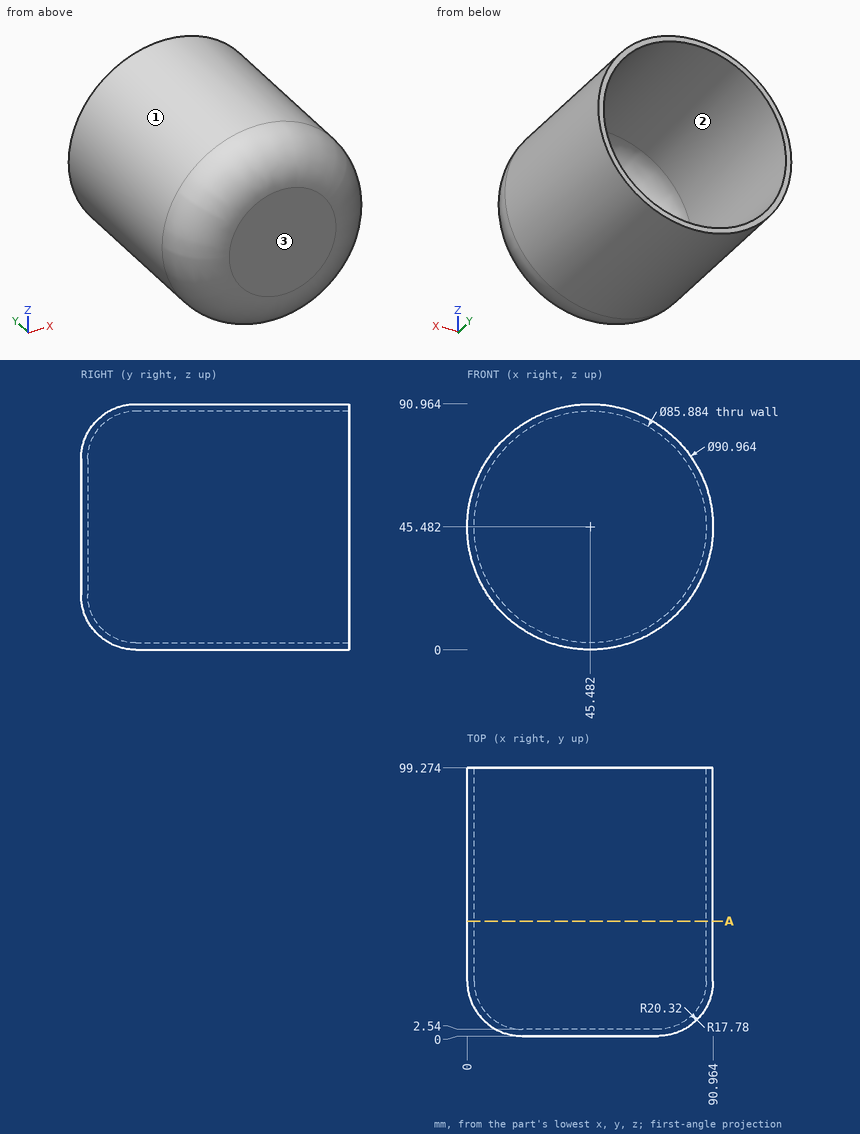
Part print with two shaded views. Sizes in mm from the minimum x, y, z corner. Round coordinates to 2 decimals unless told otherwise and drop trailing zeros. Order: outer loops, then holes, each group sorted by start corner. A loop starts at its lowest first (then second) coordinate and runs counter-clockwise, first axis right, second up. Notation, with made-up numbers: M 88,-34.75 L 105,-34.75 A17 cw 105,-12.75 Z; hole C 43,-5.5 d4. An arc over 180 degrees is marked long. Answer in a Markdown table with one row per item. Add a question column.
Q1. Wall check: L1, parallel to X at y = 28.5, z = 45; L2, parallel to X at y = 40.5, z = 19 (1 decimal); L3, parallel to Y at x = 45, z = 60.5. Give the ranges that are in metal, low to high. Write a range as from..to.
Q2. Mould opens along X. For the marked faces 1, 2 and 3 say: +X half, -X half, draft (parallel to the pull), parting line (faces both ways), or undercut.
Q3. Pin check, flat tips, straight feed: pin 1 (5 mm diameter, centred on y = 73.5, z = 10, fed in from -X) (1 decimal); pin 2 (25 mm diameter, centred on x = 54, z = 42, fed in from +Y); pin 3 (1 mm diameter, centred on x = 22, z = 27.5, fed in from -Y). Stop position of each tip, or through.
Q4. Cut at A-A on y = 42.5. Give the cut face in (x, z).
Established:
| question | item | result |
|---|---|---|
| 1 | L1 | x = 0..2.54, 88.42..90.96 |
| 1 | L2 | x = 8.5..11.7, 79.3..82.5 |
| 1 | L3 | y = 0..2.54 |
| 2 | face 1 | parting line |
| 2 | face 2 | undercut |
| 2 | face 3 | draft |
| 3 | pin 1 | stops at x = 14.2 |
| 3 | pin 2 | stops at y = 2.54 |
| 3 | pin 3 | stops at y = 0.38 |
| 4 | outline | C 45.48,45.48 d90.96; hole C 45.48,45.48 d85.88 |
